Part model, mm, in its own coordinate system. A direction names the side the tool comes from. Give positions to 0.01 mm unless a question says otherwise; leave off trailing zeros. Write each loop counter-clockwise with the first axis right and the second up, starting at its lowest first coordinate (ties: lowest second). Pieces come first, ordered by that corner, then holes. Notation, with made-up numbers: M 75,57.25 L 105,57.25 A8 cw 105,62.25 Z; hole C 35.25,71.5 d1. An arc over 180 degrees is marked long. Answer as CSV lines item,"result". Start each with the question number.
1) Slice it at B-B, the plane y = -13. Give the cut face in (x, z).
2) Wall check: line 1 along X through (y, z) = (0, 10); line 2 along X through (y, z) = (-4.5, 23); line 3 along X through (y, z) = (-16.5, 24). Give the ranges that are in metal, low to high. Write a range as from..to.
3) Slice it at A-A, the plane y = 0. Give the cut face in (x, z).
4) Tool access for faces 4 (the flat face through (14, -19.05, 13)), 5 (the cylindrical face through (-4.6, -18.2, 12.5)), 6 (the flat face through (-10.96, 9.7, 12.52)): list every direction of +Z, -Z, +X, -X, +Y, -Y with a clear straight run to the whole face (end or side of a thin tool).
5) Slice it at C-C, the plane z = 9. Give the number of separate pieces and of enclosed holes in the cut face, plus the area to 3 significant figures.
6) Pin check, flat tip, straight feed: pin 1 Ø3 at (x, z) = (0.5, 18.5) entering from -Y. Stop position of the tip, or through.
7) Mould opens along X. For faces 1 (the flat face through (9.7, 10.96, 12.52)), 2 (the cylindrical face through (18.14, -18.1, 12.52)), 3 (the flat face through (0, -4, 25.4)) say: pulls with the +X half, pulls with the -X half, needs draft (parallel to the pull), parting line crosses it, or undercut.
```python
from build123d import *

# Parameters (mm, degrees)
EXTRUDE1_DEPTH = 25.4


with BuildPart() as part:
    # Sketch1 → Extrude1 (new body)
    with BuildSketch(Plane.XY):
        with BuildLine():
            Line((2.828100791, -6.8072), (0, -6.8072))
            Line((0, -6.8072), (-2.828100791, -6.8072))
            ThreePointArc((-2.828100791, -6.8072), (-4.154656747, -7.029801128), (-5.335891418, -7.673219048))
            ThreePointArc((-5.335891418, -7.673219048), (-7.314841404, -9.397406099), (-9.105295238, -11.316608824))
            ThreePointArc((-9.105295238, -11.316608824), (-9.812696364, -12.53999053), (-10.0584, -13.931647412))
            Line((-10.0584, -13.931647412), (-10.0584, -15.614648356))
            ThreePointArc((-10.0584, -15.614648356), (-8.91004969, -16.763999564), (-7.759698458, -15.616651022))
            ThreePointArc((-7.759698458, -15.616651022), (-7.475165883, -14.913287543), (-6.782702014, -14.603170209))
            Line((-6.782702014, -14.603170209), (-5.055502014, -14.536817878))
            ThreePointArc((-5.055502014, -14.536817878), (-4.312003742, -14.819989072), (-4.0005, -15.552069001))
            Line((-4.0005, -15.552069001), (-4.0005, -16.760361628))
            ThreePointArc((-4.0005, -16.760361628), (-4.568340141, -18.169354143), (-5.954495972, -18.790863874))
            Line((-5.954495972, -18.790863874), (-12.7, -19.05))
            Line((-12.7, -19.05), (-15.875, -19.05))
            ThreePointArc((-15.875, -19.05), (-18.12006403, -18.12006403), (-19.05, -15.875))
            Line((-19.05, -15.875), (-19.05, 15.875))
            ThreePointArc((-19.05, 15.875), (-18.12006403, 18.12006403), (-15.875, 19.05))
            Line((-15.875, 19.05), (0, 19.05))
            Line((0, 19.05), (15.875, 19.05))
            ThreePointArc((15.875, 19.05), (18.12006403, 18.12006403), (19.05, 15.875))
            Line((19.05, 15.875), (19.05, -15.875))
            ThreePointArc((19.05, -15.875), (18.12006403, -18.12006403), (15.875, -19.05))
            Line((15.875, -19.05), (12.7, -19.05))
            Line((12.7, -19.05), (5.954495972, -18.790863874))
            ThreePointArc((5.954495972, -18.790863874), (4.568340141, -18.169354143), (4.0005, -16.760361628))
            Line((4.0005, -16.760361628), (4.0005, -15.552069001))
            ThreePointArc((4.0005, -15.552069001), (4.312003742, -14.819989072), (5.055502014, -14.536817878))
            Line((5.055502014, -14.536817878), (6.782702014, -14.603170209))
            ThreePointArc((6.782702014, -14.603170209), (7.475165883, -14.913287543), (7.759698458, -15.616651022))
            ThreePointArc((7.759698458, -15.616651022), (8.91004969, -16.763999564), (10.0584, -15.614648356))
            Line((10.0584, -15.614648356), (10.0584, -13.931647412))
            ThreePointArc((10.0584, -13.931647412), (9.812696364, -12.53999053), (9.105295238, -11.316608824))
            ThreePointArc((9.105295238, -11.316608824), (7.314841404, -9.397406099), (5.335891418, -7.673219048))
            ThreePointArc((5.335891418, -7.673219048), (4.154656747, -7.029801128), (2.828100791, -6.8072))
        make_face()
        with BuildLine():
            Line((4.191663684, 5.448899541), (15.364356459, 16.621592316))
            ThreePointArc((15.364356459, 16.621592316), (15.446946878, 17.036802388), (15.094948776, 17.272))
            Line((15.094948776, 17.272), (0, 17.272))
            Line((0, 17.272), (-15.094948776, 17.272))
            ThreePointArc((-15.094948776, 17.272), (-15.446946878, 17.036802388), (-15.364356459, 16.621592316))
            Line((-15.364356459, 16.621592316), (-4.191663684, 5.448899541))
            ThreePointArc((-4.191663684, 5.448899541), (-3.957294594, 5.338921804), (-3.706747429, 5.40411452))
            ThreePointArc((-3.706747429, 5.40411452), (-1.940384881, 6.259339962), (0, 6.5532))
            ThreePointArc((0, 6.5532), (1.940384881, 6.259339962), (3.706747429, 5.40411452))
            ThreePointArc((3.706747429, 5.40411452), (3.957294594, 5.338921804), (4.191663684, 5.448899541))
        make_face(mode=Mode.SUBTRACT)
        with BuildLine():
            Line((-17.272, 15.094948776), (-17.272, -15.621))
            ThreePointArc((-17.272, -15.621), (-16.788433296, -16.788433296), (-15.621, -17.272))
            Line((-15.621, -17.272), (-12.4714, -17.272))
            ThreePointArc((-12.4714, -17.272), (-12.201992316, -17.160407684), (-12.0904, -16.891))
            Line((-12.0904, -16.891), (-12.0904, -13.931647412))
            ThreePointArc((-12.0904, -13.931647412), (-11.721844546, -11.84416209), (-10.660742857, -10.00908953))
            ThreePointArc((-10.660742857, -10.00908953), (-8.000870719, -7.259428949), (-4.984332303, -4.906547928))
            ThreePointArc((-4.984332303, -4.906547928), (-4.819224111, -4.638901343), (-4.91158257, -4.338293085))
            ThreePointArc((-4.91158257, -4.338293085), (-6.540953358, -0.40044901), (-5.40411452, 3.706747429))
            ThreePointArc((-5.40411452, 3.706747429), (-5.338921804, 3.957294594), (-5.448899541, 4.191663684))
            Line((-5.448899541, 4.191663684), (-16.621592316, 15.364356459))
            ThreePointArc((-16.621592316, 15.364356459), (-17.036802388, 15.446946878), (-17.272, 15.094948776))
        make_face(mode=Mode.SUBTRACT)
        with BuildLine():
            Line((17.272, 15.094948776), (17.272, -15.621))
            ThreePointArc((17.272, -15.621), (16.788433296, -16.788433296), (15.621, -17.272))
            Line((15.621, -17.272), (12.4714, -17.272))
            ThreePointArc((12.4714, -17.272), (12.201992316, -17.160407684), (12.0904, -16.891))
            Line((12.0904, -16.891), (12.0904, -13.931647412))
            ThreePointArc((12.0904, -13.931647412), (11.721844546, -11.84416209), (10.660742857, -10.00908953))
            ThreePointArc((10.660742857, -10.00908953), (8.000870719, -7.259428949), (4.984332303, -4.906547928))
            ThreePointArc((4.984332303, -4.906547928), (4.819224111, -4.638901343), (4.91158257, -4.338293085))
            ThreePointArc((4.91158257, -4.338293085), (6.540953358, -0.40044901), (5.40411452, 3.706747429))
            ThreePointArc((5.40411452, 3.706747429), (5.338921804, 3.957294594), (5.448899541, 4.191663684))
            Line((5.448899541, 4.191663684), (16.621592316, 15.364356459))
            ThreePointArc((16.621592316, 15.364356459), (17.036802388, 15.446946878), (17.272, 15.094948776))
        make_face(mode=Mode.SUBTRACT)
        with BuildLine():
            ThreePointArc((0, 3.302), (-3.302, 0), (0, -3.302))
            ThreePointArc((0, -3.302), (3.302, 0), (0, 3.302))
        make_face(mode=Mode.SUBTRACT)
    extrude(amount=EXTRUDE1_DEPTH)


solid = part.part
```
Found:
1,outline,"M -19.05,0 L -17.27,0 L -17.27,25.4 L -19.05,25.4 Z; M -12.02,0 L -9.95,0 L -9.95,25.4 L -12.02,25.4 Z; M 9.95,0 L 12.02,0 L 12.02,25.4 L 9.95,25.4 Z; M 17.27,0 L 19.05,0 L 19.05,25.4 L 17.27,25.4 Z"
2,line 1,"-19.05..-17.27, -6.55..-3.3, 3.3..6.55, 17.27..19.05"
2,line 2,"-19.05..-17.27, -4.83..4.83, 17.27..19.05"
2,line 3,"-18.99..-17.02, -12.09..-9.64, -8.18..-4, 4..8.18, 9.64..12.09, 17.02..18.99"
3,outline,"M -19.05,0 L -17.27,0 L -17.27,25.4 L -19.05,25.4 Z; M -6.55,0 L -3.3,0 L -3.3,25.4 L -6.55,25.4 Z; M 3.3,0 L 6.55,0 L 6.55,25.4 L 3.3,25.4 Z; M 17.27,0 L 19.05,0 L 19.05,25.4 L 17.27,25.4 Z"
4,face 4,"+Z, -Z, +X, -X, -Y"
4,face 5,"+Z, -Z, -Y"
4,face 6,"+Z, -Z"
5,separate pieces,"1"
5,enclosed holes,"4"
5,area,"484 mm²"
6,pin 1,"y = -6.81"
7,face 1,"undercut"
7,face 2,"pulls with the +X half"
7,face 3,"needs draft"
